Can you work these out from the model? Positions are in its coordinate system, mm. A direction names the side the tool comes from. Round coordinates to 2 decimals unless told otherwise and drop trailing zeros. Loops run counter-clockwise (first coordinate to the right, second up) from the corner with the lowest first, then second, coordinate; pieces in that order, holes last.
Autodesk Inventor part; units mm, degrees
ref_plane "YZ Plane" through (0, 0, 0) normal (1, 0, 0) x (0, 1, 0)
ref_plane "XZ Plane" through (0, 0, 0) normal (0, 1, 0) x (-1, 0, 0)
ref_plane "XY Plane" through (0, 0, 0) normal (0, 0, 1) x (1, 0, 0)
sketch "Sketch1" plane through (0, 0, 0) normal (0, 0, 1) x (1, 0, 0)
  line L0 (19.05, -19.05) -> (-19.05, -19.05)
  line L1 (-19.05, -19.05) -> (-19.05, 19.05)
  line L2 (-19.05, 19.05) -> (19.05, 19.05)
  line L3 (19.05, 19.05) -> (19.05, -19.05)
  point P0 (0, 0)
  point P1 (-19.05, 0)
  point P2 (0, 19.05)
  dimension "d0" = 38.1
  dimension "d1" = 38.1
extrude "Extrusion1" add sketch "Sketch1" along normal blind 6.35
sketch "Sketch2" plane through (0, 0, 6.35) normal (0, 0, 1) x (1, 0, 0)
  line L0 (-19.05, -19.05) -> (-19.05, 19.05)
  line L1 (-19.05, 19.05) -> (19.05, 19.05)
  line L2 (8.636, -8.255) -> (-8.636, -8.255)
  line L3 (-8.636, -8.255) -> (-8.636, 8.255)
  line L4 (-8.636, 8.255) -> (8.636, 8.255)
  line L5 (8.636, 8.255) -> (8.636, -8.255)
  point P0 (0, 0)
  point P1 (0, 8.255)
  point P2 (0, 19.05)
  point P3 (-8.636, 0)
  point P4 (-19.05, 0)
  dimension "d4" = 17.272
  dimension "d5" = 16.51
extrude "Extrusion2" add sketch "Sketch2" along normal blind 6.858
sketch "Sketch3" plane through (0, 0, 13.208) normal (0, 0, 1) x (1, 0, 0)
  circle A0 centre (0, 0) radius 7.493
  point P0 (0, 0)
  dimension "d8" = 14.986
extrude "Extrusion3" add sketch "Sketch3" along normal blind 17.272
properties part number "Camera - SONY CCD"
(1) For pin 1 (1 mm diameter, centred on x = -1.5, z = 14, fed in from +Y); pin 2 (2 mm diameter, centred on x = -2.5, y = -11, fed in from -Z); pin 3 (2 mm diameter, centred on y = -3, z = 11, fed in from -X); pin 4 (5.5 mm diameter, centred on x = 1.5, z = 9.5, fed in from -Y) (3 decimals), each with a flat end and sliding along its axis, tell me the tip position at first contact or that it passes through.
(2) Suppose I cut it at C-C (z = 19). Write out the boundary of the cut face in (x, y), then the cut area to 3 significant figures.
(3) If I drill on line 1 (Z direction, x = -6.5, y = -7); line 2 (Z direction, x = -14, y = -9.5); line 3 (Y direction, x = -0.5, z = 9) (3 decimals), over which ranges is the centre line in solid material (lowest first)?
(4) Suppose I cut it at B-B (y = 0). Write out the boundary of the cut face in (x, z), then the cut area to 3 significant figures.
(5) Suppose I cut it at D-D (y = -9). Write out the boundary of the cut face in (x, z).
(6) Suppose I cut it at A-A (x = 0). Write out the boundary of the cut face in (y, z) (3 decimals).
(7) We'd pull the mould along Y, two halves only. Please class faces 1 (the flat face through (0, 8.255, 10)), 2 (the flat face through (0, -19.05, 3)), 3 (the flat face through (-19.05, 0, 3)): released by +Y, released by -Y, zero draft, split by the parting line, or undercut.
(8) Which directions (+Z, -Z, +X, -X, +Y, -Y) give clear straight access to the entire face, cutting with the end or side of a thin tool? Please do faces 4 (the flat face through (0, -8.255, 10)), 5 (the flat face through (-8.636, 0, 10)), 6 (the flat face through (8.636, 0, 10)).
Check result:
1. pin 1: stops at y = 7.43
1. pin 2: stops at z = 0
1. pin 3: stops at x = -8.64
1. pin 4: stops at y = -8.255
2. outline: circle Ø14.99 at (0, 0)
2. area: 176 mm2
3. line 1: z = 0 to 13.21
3. line 2: z = 0 to 6.35
3. line 3: y = -8.255 to 8.255
4. outline: (-19.05, 0) - (19.05, 0) - (19.05, 6.35) - (8.64, 6.35) - (8.64, 13.21) - (7.49, 13.21) - (7.49, 30.48) - (-7.49, 30.48) - (-7.49, 13.21) - (-8.64, 13.21) - (-8.64, 6.35) - (-19.05, 6.35) - close
4. area: 619 mm2
5. outline: (-19.05, 0) - (19.05, 0) - (19.05, 6.35) - (-19.05, 6.35) - close
6. outline: (-19.05, 0) - (19.05, 0) - (19.05, 6.35) - (8.255, 6.35) - (8.255, 13.208) - (7.493, 13.208) - (7.493, 30.48) - (-7.493, 30.48) - (-7.493, 13.208) - (-8.255, 13.208) - (-8.255, 6.35) - (-19.05, 6.35) - close
7. face 1: released by +Y
7. face 2: released by -Y
7. face 3: zero draft
8. face 4: +Z, +X, -X, -Y
8. face 5: +Z, -X, +Y, -Y
8. face 6: +Z, +X, +Y, -Y
